Could you check a few things on this drawing? It's one solid part, dimensions in mm from its lowest x, y, z. A direction names the side the tool comes from. Coordinates: 2 decimals unless noted, no trailing zeros. Write each loop counter-clockwise with the first axis right and the second up, starting at its lowest first coordinate (ties: lowest second). Pieces come first, ordered by that corner, then holes.
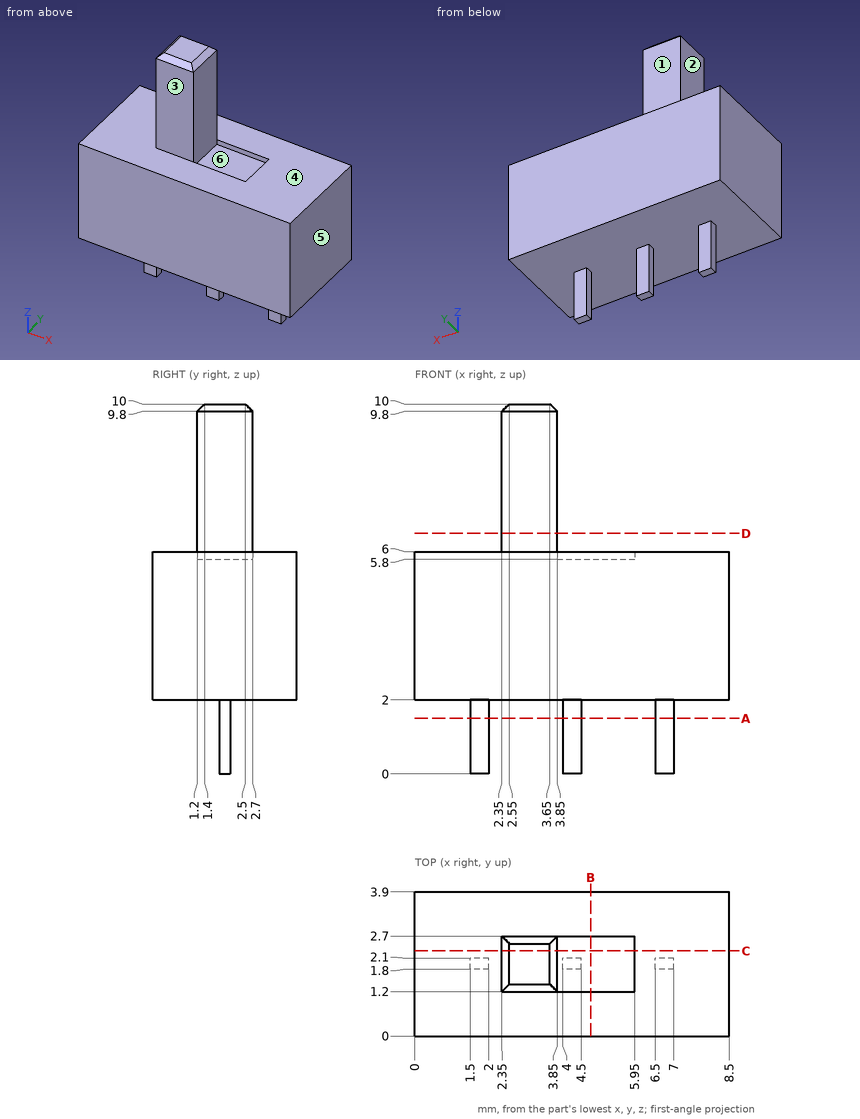
1) I need wall thicknesses on probe 1 along Z at (x, y) = (6.5, 2.3); probe 2 along X at (y, z) = (2.2, 8.25); probe 3 along Z at (x, y) = (4.25, 1.95). Which ranges of each line are inside material? Lowest first, please.
Values follow:
probe 1: z = 2 to 6
probe 2: x = 2.35 to 3.85
probe 3: z = 0 to 5.8
2) On a 3-axis mill with a long thin cutter (end or side, diameter ignored), from which of +Z, -Z, +X, -X, +Y, -Y can I reach the whole of each face in a straight line? I mean the marked faces 1, 2 and 3. Say none if no direction works.
Values follow:
face 1: +Z, +X, -X, +Y
face 2: +Z, -X, +Y, -Y
face 3: +Z, +X, -X, -Y
3) We'd pull the mould along X, two halves only. Please class the marked faces 4, 5 and 6: pulls with the +X half, pulls with the -X half, needs draft (parallel to the pull), parting line crosses it, or undercut.
Values follow:
face 4: needs draft
face 5: pulls with the +X half
face 6: undercut
4) Imagine slicing it at D-D on z = 6.5. Please give me the cut outline in (x, y).
Values follow:
outline: (2.35, 1.2) - (3.85, 1.2) - (3.85, 2.7) - (2.35, 2.7) - close
5) Imagine slicing it at C-C on y = 2.3. Please give me the cut outline in (x, z).
Values follow:
outline: (0, 2) - (8.5, 2) - (8.5, 6) - (5.95, 6) - (5.95, 5.8) - (3.85, 5.8) - (3.85, 9.8) - (3.65, 10) - (2.55, 10) - (2.35, 9.8) - (2.35, 6) - (0, 6) - close
6) Will these pins go through, and if not, where does the flat tip stop? pin 1 (0.6 mm diameter, centred on x = 1.5, z = 0.5, fed in from +Y); pin 2 (1 mm diameter, centred on x = 6, y = 3, fed in from +Z); pin 3 (1.6 mm diameter, centred on x = 3, z = 8.5, fed in from -Y); pin 4 (1.2 mm diameter, centred on x = 2.5, y = 2.5, fed in from +Z).
Values follow:
pin 1: stops at y = 2.1
pin 2: stops at z = 6
pin 3: stops at y = 1.2
pin 4: stops at z = 10
7) Imagine slicing it at A-A on z = 1.5. Please give me the cut outline in (x, y), then the cut area to 3 significant figures.
Values follow:
outline: (1.5, 1.8) - (2, 1.8) - (2, 2.1) - (1.5, 2.1) - close; (4, 1.8) - (4.5, 1.8) - (4.5, 2.1) - (4, 2.1) - close; (6.5, 1.8) - (7, 1.8) - (7, 2.1) - (6.5, 2.1) - close
area: 0.450 mm2
8) Imagine slicing it at B-B on x = 4.75. Please give me the cut outline in (y, z), then the cut area to 3 significant figures.
Values follow:
outline: (0, 2) - (3.9, 2) - (3.9, 6) - (2.7, 6) - (2.7, 5.8) - (1.2, 5.8) - (1.2, 6) - (0, 6) - close
area: 15.3 mm2
